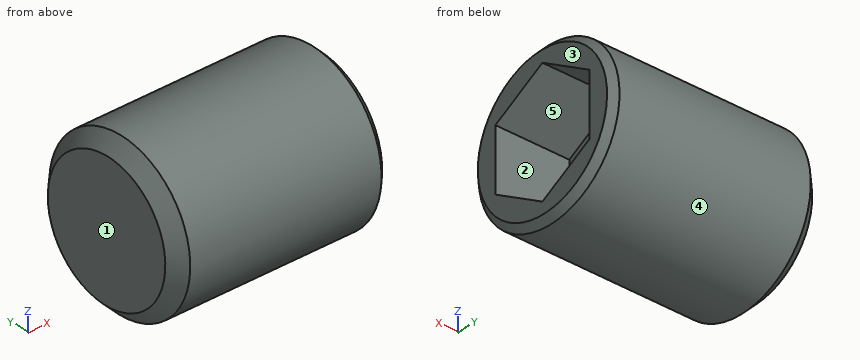
```python
from build123d import *

# Parameters (mm, degrees)
ESQUISSE1_W             = 8
ESQUISSE1_H             = 3
CHANFREIN2_SIZE         = 0.5
EMPREINTE_POUR_CL_DEPTH = 2.8
CHANFREIN3_SIZE         = 0.25


with BuildPart() as part:
    # Esquisse1 → Base-Révolution (revolve)
    with BuildSketch(Plane.XY, mode=Mode.PRIVATE) as base_r_volution_sk:
        with Locations((4, 1.5)):
            Rectangle(ESQUISSE1_W, ESQUISSE1_H)
    revolve(base_r_volution_sk.sketch.rotate(Axis((-25.828475034, 0, 0), (1, 0, 0)), 90), axis=Axis((-25.828475034, 0, 0), (1, 0, 0)))

    # Chanfrein2
    chanfrein2_edges = [part.edges().sort_by_distance(p)[0] for p in [
        (0, 0, -3),
    ]]
    chamfer(chanfrein2_edges, length=CHANFREIN2_SIZE)

    # Esquisse2 → Empreinte pour clé (cut)
    with BuildSketch(Plane(origin=(8, 0, 0), x_dir=(0, 0, -1), z_dir=(1, 0, 0))):
        Polygon((2.309401077, 0), (1.154700538, 2), (-1.154700538, 2), (-2.309401077, 0), (-1.154700538, -2), (1.154700538, -2), align=None)
    extrude(amount=-EMPREINTE_POUR_CL_DEPTH, mode=Mode.SUBTRACT)

    # Chanfrein3
    chanfrein3_edges = [part.edges().sort_by_distance(p)[0] for p in [
        (8, 0, -3),
    ]]
    chamfer(chanfrein3_edges, length=CHANFREIN3_SIZE)


solid = part.part
```
For this review, take the finished solid that the model builds, in its own axes (mm). Face numbers are marked on the shaded views. A direction names the side the tool comes from. Coordinates: 2 decimals unless noted, no trailing zeros. Write each loop counter-clockwise with the first axis right and the second up, starting at its lowest first coordinate (ties: lowest second). Pieces come first, ordered by that corner, then holes.
(1) For pin 1 Ø2 at (x, y) = (3.5, -1.5) entering from -Z; pin 2 Ø1.5 at (x, y) = (6.5, -1.5) entering from +Z; pin 3 Ø2 at (x, y) = (4, 2) entering from -Z, all flat-tipped, find the tip position at first contact; note any pin that passes through.
(2) The part is to be moulded in two halves that separate along Z. For the marked faces 3, 4 and 5, say which applies: +Z half, -Z half, draft (parallel to the pull), parting line (faces both ways), or undercut.
(3) Add section A-A on z = 0. Give the boundary of the cut face in (x, y), then the cut area to 3 significant figures.
(4) Tool access review of the marked faces 1 and 2: name each direction out of +Z, -Z, +X, -X, +Y, -Y from which nothing blocks a thin tool from reaching the whole face with its end or side.
(5) Wall thickness on probe 1 along Z at (x, y) = (3.5, 1.2); probe 2 along X at (y, z) = (1.25, -1.4); probe 3 along Y at (x, z) = (6, -1.05): over which ranges is each line inside the solid? List them lowest first.
(6) Add section B-B on x = 1.75. Give the boundary of the cut face in (y, z).
Answer sheet:
1. pin 1: stops at z = -2.96
1. pin 2: stops at z = 2.9
1. pin 3: stops at z = -2.83
2. face 3: draft
2. face 4: parting line
2. face 5: undercut
3. outline: (0, -2.5) - (0.5, -3) - (7.75, -3) - (8, -2.75) - (8, -2) - (5.2, -2) - (5.2, 2) - (8, 2) - (8, 2.75) - (7.75, 3) - (0.5, 3) - (0, 2.5) - close
3. area: 36.5 mm2
4. face 1: +Z, -Z, -X, +Y, -Y
4. face 2: +X
5. probe 1: z = -2.75 to 2.75
5. probe 2: x = 0 to 5.2
5. probe 3: y = -2.81 to -2, 2 to 2.81
6. outline: circle Ø6 at (0, 0)
